Input: part model. Units: mm. Frame: model coordinates. Face numbers are marked on the shaded views. A direction names the side the tool comes from. Give positions to 0.01 mm unless a question says otherwise; leave off trailing zeros. Loops run counter-clockwise (first coordinate to the right, second up) from the corner with the lowest first, then second, coordinate; pieces in that order, holes last. Notation, with made-up numbers: (55.5, 72) -> (85.5, 72) arc R29 ccw to (85.5, 101) -> close; hole circle Ø11 at (-5, -20.75). An arc over 180 degrees is marked (long way). Answer as a JSON object with one key per item and string values. Group by question number.
```python
from build123d import *

# Parameters (mm, degrees)
F0_W      = 84.25
F0_H      = 59.75
F0_W_2    = 76.25
F0_H_2    = 51.75
F1_DEPTH  = 14
F2_W      = 80.25
F2_H      = 55.75
F3_DEPTH  = 10
F5_DEPTH  = 62
F6_W      = 12.75
F6_H      = 2.75
F7_DEPTH  = 2
F8_R      = 2.375
F9_DEPTH  = 0.25
F10_W     = 84.25
F10_H     = 59.75
F10_W_2   = 82.25
F10_H_2   = 57.75
F11_DEPTH = 3
F12_W     = 7.5
F12_H     = 2
F13_DEPTH = 85
F14_R     = 1
F15_R     = 2.25
F16_DEPTH = 2.54
F17_R     = 1.125
F18_DEPTH = 4
F19_DEPTH = 2.54
F20_R     = 1.125
F21_DEPTH = 4


with BuildPart() as f1:
    # F0 (on Top) → F1 (new body)
    with BuildSketch(Plane.XY):
        Rectangle(F0_W, F0_H)
        Rectangle(F0_W_2, F0_H_2, mode=Mode.SUBTRACT)
        Rectangle(F0_W_2, F0_H_2)
    extrude(amount=F1_DEPTH)

    # F2 (on face) → F3 (cut)
    with BuildSketch(Plane.XY.offset(14)):
        Rectangle(F2_W, F2_H)
    extrude(amount=-F3_DEPTH, mode=Mode.SUBTRACT)

    # F4 (on face) → F5 (cut)
    with BuildSketch(Plane.XZ.offset(29.875)):
        Polygon((-4.375, 0), (0, 0), (0, 2), (-6.25, 2), (-6.25, 1), (-4.375, 1), align=None)
        Polygon((0, 2), (0, 0), (4.375, 0), (4.375, 1), (6.25, 1), (6.25, 2), align=None)
    extrude(amount=-F5_DEPTH, mode=Mode.SUBTRACT)

    # F6 (on Top) → F7 (cut)
    with BuildSketch(Plane.XY):
        with Locations((0, 29.875)):
            Rectangle(F6_W, F6_H)
        with Locations((0, 14.9375)):
            Rectangle(F6_W, F6_H)
        Rectangle(F6_W, F6_H)
        with Locations((0, -14.9375)):
            Rectangle(F6_W, F6_H)
        with Locations((0, -29.875)):
            Rectangle(F6_W, F6_H)
    extrude(amount=F7_DEPTH, mode=Mode.SUBTRACT)

    # F8 (on face) → F9 (join)
    with BuildSketch(Plane(origin=(0, 0, 2), x_dir=(1, 0, 0), z_dir=(0, 0, -1))):
        with Locations((0, 25.125)):
            Circle(F8_R)
        with Locations((0, 8.375)):
            Circle(F8_R)
        with Locations((0, -8.375)):
            Circle(F8_R)
        with Locations((0, -25.125)):
            Circle(F8_R)
    extrude(amount=F9_DEPTH)

    # F10 (on face) → F11 (cut)
    with BuildSketch(Plane.XY.offset(14)):
        Rectangle(F10_W, F10_H)
        Rectangle(F10_W_2, F10_H_2, mode=Mode.SUBTRACT)
    extrude(amount=-F11_DEPTH, mode=Mode.SUBTRACT)

    # F12 (on face) → F13 (cut)
    with BuildSketch(Plane.YZ.offset(42.125)):
        with Locations((0, 8)):
            Rectangle(F12_W, F12_H)
    extrude(amount=-F13_DEPTH, mode=Mode.SUBTRACT)

    # F14
    f14_edges = [f1.edges().sort_by_distance(p)[0] for p in [
        (24.25, -29.875, 0),
        (42.125, 0, 0),
        (24.25, 29.875, 0),
        (-24.25, 29.875, 0),
        (-42.125, 0, 0),
        (-24.25, -29.875, 0),
        (42.125, -29.875, 5.5),
        (42.125, 29.875, 5.5),
        (-42.125, -29.875, 5.5),
        (-42.125, 29.875, 5.5),
    ]]
    fillet(f14_edges, radius=F14_R)

    # F15 (on face) → F16 (join)
    with BuildSketch(Plane.XY.offset(4)):
        with Locations((-33.625, 20.375)):
            Circle(F15_R)
    extrude(amount=F16_DEPTH)

    # F17 (on face) → F18 (join)
    with BuildSketch(Plane.XY.offset(6.54)):
        with Locations((-33.625, 20.375)):
            Circle(F17_R)
    extrude(amount=F18_DEPTH)

    # F15 (on face) → F19 (join)
    with BuildSketch(Plane.XY.offset(4)):
        with Locations((33.125, -21.875)):
            Circle(F15_R)
    extrude(amount=F19_DEPTH)

    # F20 (on face) → F21 (join)
    with BuildSketch(Plane.XY.offset(6.54)):
        with Locations((33.125, -21.875)):
            Circle(F20_R)
    extrude(amount=F21_DEPTH)


solid = f1.part
```
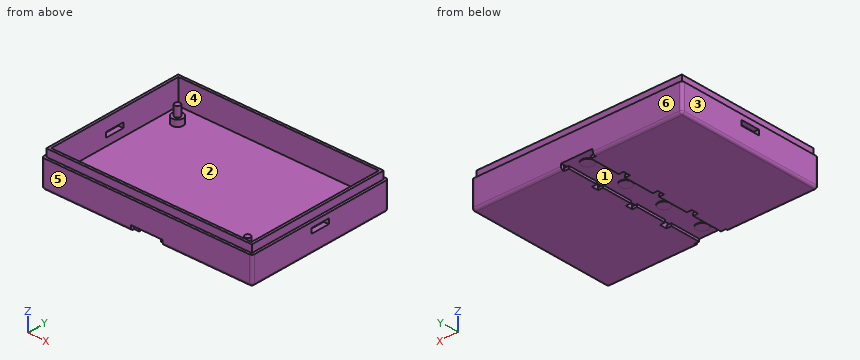
Q1. Pull-direction query (Y, two-part tool) for the marked faces 4, 5 and 6; classes: +Y half, -Y half, draft (parallel to the pull), parting line (faces both ways), or undercut.
Q2. Section A-A on z = 12.75. Return the cut outline in (x, y) (3 decimals), then the cut area to 3 significant figures.
Q3. Section B-B on x = 0. Return the cut outline in (y, z) (3 decimals), then the cut area to 3 significant figures.
Q4. Section C-C on x = 28.5. Return the cut outline in (y, z) (3 decimals).
Q5. Set-up query: the marked faces 1, 2 and 3. Return all of +Z, -Z, +X, -X, +Y, -Y with unobstructed straight access to the full face (end or side cutting, diameter ignored); none if empty.
Q6. Ray query, probe 1 along Y at (x, z) = (-35.5, 11.5) (3 decimals); probe 2 along X at (y, z) = (5.5, 8.75) (3 decimals); probe 3 along X at (y, z) = (22, 6.25) (3 decimals). Return the intervals inside material, ascending.
Q7. Pin query (flat end, axial travel): pin 1 Ø6 at (x, y) = (-30.5, -17) entering from +Z; pin 2 Ø2.5 at (x, y) = (-1, -8.5) entering from -Z; pin 3 Ø1 at (x, z) = (-5.5, 0.5) entering from -Y. Return the tip coordinate at first contact, or that it passes through.
Numbers:
{
 "1": {"face 4": "undercut", "face 5": "-Y half", "face 6": "+Y half"},
 "2": {"outline": "(-41.125, -28.875) -> (41.125, -28.875) -> (41.125, 28.875) -> (-41.125, 28.875) -> close; hole (-40.125, -27.875) -> (40.125, -27.875) -> (40.125, 27.875) -> (-40.125, 27.875) -> close", "area": "276 mm²"},
 "3": {"outline": "(-29.875, 2) -> (-27.5, 2) -> (-27.5, 1.75) -> (-22.75, 1.75) -> (-22.75, 2) -> (-10.75, 2) -> (-10.75, 1.75) -> (-6, 1.75) -> (-6, 2) -> (6, 2) -> (6, 1.75) -> (10.75, 1.75) -> (10.75, 2) -> (22.75, 2) -> (22.75, 1.75) -> (27.5, 1.75) -> (27.5, 2) -> (29.875, 2) -> (29.875, 11) -> (28.875, 11) -> (28.875, 14) -> (27.875, 14) -> (27.875, 4) -> (-27.875, 4) -> (-27.875, 14) -> (-28.875, 14) -> (-28.875, 11) -> (-29.875, 11) -> close", "area": "158 mm²"},
 "4": {"outline": "(-29.875, 1) arc R1 ccw to (-28.875, 0) -> (28.875, 0) arc R1 ccw to (29.875, 1) -> (29.875, 11) -> (28.875, 11) -> (28.875, 14) -> (27.875, 14) -> (27.875, 4) -> (-27.875, 4) -> (-27.875, 14) -> (-28.875, 14) -> (-28.875, 11) -> (-29.875, 11) -> close"},
 "5": {"face 1": "none", "face 2": "+Z", "face 3": "+Z, -Z, -X, +Y, -Y"},
 "6": {"probe 1": "y = -28.875 to -27.875, 27.875 to 28.875", "probe 2": "x = -42.125 to -40.125, 40.125 to 42.125", "probe 3": "x = -42.125 to -40.125, -35.181 to -32.069, 40.125 to 42.125"},
 "7": {"pin 1": "stops at z = 4", "pin 2": "stops at z = 1.75", "pin 3": "stops at y = -28.5"}
}
